```python
from build123d import *

# Parameters (mm, degrees)
SKETCH1_W                  = 600
SKETCH1_H                  = 500
BOSS_EXTRUDE1_DEPTH        = 226
SKETCH2_OUTSIDE_W          = 764.614
SKETCH2_OUTSIDE_H          = 664.614
CUT_EXTRUDE1_DEPTH         = 452.193971591
CUT_EXTRUDE8_DEPTH         = 452.193971591
CUT_EXTRUDE2_DEPTH         = 689.168583997
CUT_EXTRUDE3_DEPTH         = 689.168583997
SKETCH7_R                  = 2.5
CUT_EXTRUDE5_DEPTH         = 25
SKETCH8_R                  = 9.525
CUT_EXTRUDE6_DEPTH         = 35
F_6_0MM_DOWEL_HOLE1_D      = 6
F_6_0MM_DOWEL_HOLE1_DEPTH  = 28.197418143
F_6_0MM_DOWEL_HOLE1_TIP    = 1.802581857
F_6_0MM_DOWEL_HOLE2_D      = 6
F_6_0MM_DOWEL_HOLE2_DEPTH  = 28.197418143
F_6_0MM_DOWEL_HOLE2_TIP    = 1.802581857
F_6_0MM_DOWEL_HOLE3_D      = 6
F_6_0MM_DOWEL_HOLE3_DEPTH  = 28.197418143
F_6_0MM_DOWEL_HOLE3_TIP    = 1.802581857
FILLET2_R                  = 30
F_10_0MM_DOWEL_HOLE1_D     = 10
F_10_0MM_DOWEL_HOLE1_DEPTH = 28
F_10_0MM_DOWEL_HOLE1_TIP   = 3.004303095
CUT_EXTRUDE9_DEPTH         = 35
CHAMFER1_SIZE              = 6
CHAMFER1_SIZE_2            = 114.486820126
CHAMFER2_SIZE              = 3
CHAMFER2_SIZE_2            = 171.477335318
CHAMFER2_SIZE_3            = 42.90199877
CHAMFER3_SIZE              = 3
CHAMFER3_SIZE_2            = 171.477335318
CHAMFER3_SIZE_3            = 42.90199877
FILLET3_R                  = 8


with BuildPart() as part:
    # Sketch1 → Boss-Extrude1 (new body)
    with BuildSketch(Plane.XY):
        Rectangle(SKETCH1_W, SKETCH1_H)
    extrude(amount=BOSS_EXTRUDE1_DEPTH)

    # Sketch2 outside → Cut-Extrude1 (cut, through all)
    with BuildSketch(Plane.XY.offset(226)):
        Rectangle(SKETCH2_OUTSIDE_W, SKETCH2_OUTSIDE_H)
        Polygon((-210, -250), (-210, -225), (-210, -30), (210, -30), (210, -225), (210, -250), (300, -250), (300, 250), (-300, 250), (-300, -250), align=None, mode=Mode.SUBTRACT)
    extrude(amount=-CUT_EXTRUDE1_DEPTH, mode=Mode.SUBTRACT)

    # Sketch22 → Cut-Extrude8 (cut, through all)
    with BuildSketch(Plane.XY.offset(226)):
        Polygon((-210, -30), (210, -30), (105, 5), (0, 5), (-105, 5), align=None)
    extrude(amount=-CUT_EXTRUDE8_DEPTH, mode=Mode.SUBTRACT)

    # Sketch4 → Cut-Extrude2 (cut, through all)
    with BuildSketch(Plane.ZY.offset(300)):
        Polygon((148, 25), (148, 5), (226, -200), (226, -165), (226, -145), (226, 250), (148, 250), align=None)
    extrude(amount=-CUT_EXTRUDE2_DEPTH, mode=Mode.SUBTRACT)

    # Sketch5 → Cut-Extrude3 (cut, through all)
    with BuildSketch(Plane.ZY.offset(300)):
        Polygon((131, 160), (131, 165), (148, 185), (148, 65), (131, 85), (131, 90), (131, 125), align=None)
    extrude(amount=-CUT_EXTRUDE3_DEPTH, mode=Mode.SUBTRACT)

    # Sketch7 → Cut-Extrude5 (cut)
    with BuildSketch(Plane.XY.offset(148)):
        with Locations((-270, 215)):
            Circle(SKETCH7_R)
        with Locations((-210, 215)):
            Circle(SKETCH7_R)
        with Locations((-150, 215)):
            Circle(SKETCH7_R)
        with Locations((-90, 215)):
            Circle(SKETCH7_R)
        with Locations((-30, 215)):
            Circle(SKETCH7_R)
        with Locations((30, 215)):
            Circle(SKETCH7_R)
        with Locations((90, 215)):
            Circle(SKETCH7_R)
        with Locations((150, 215)):
            Circle(SKETCH7_R)
        with Locations((210, 215)):
            Circle(SKETCH7_R)
        with Locations((270, 215)):
            Circle(SKETCH7_R)
        with Locations((-210, 35)):
            Circle(SKETCH7_R)
        with Locations((-150, 35)):
            Circle(SKETCH7_R)
        with Locations((-90, 35)):
            Circle(SKETCH7_R)
        with Locations((-30, 35)):
            Circle(SKETCH7_R)
        with Locations((30, 35)):
            Circle(SKETCH7_R)
        with Locations((90, 35)):
            Circle(SKETCH7_R)
        with Locations((150, 35)):
            Circle(SKETCH7_R)
        with Locations((210, 35)):
            Circle(SKETCH7_R)
        with Locations((270, 35)):
            Circle(SKETCH7_R)
        with Locations((-270, 35)):
            Circle(SKETCH7_R)
    extrude(amount=-CUT_EXTRUDE5_DEPTH, mode=Mode.SUBTRACT)

    # Sketch8 → Cut-Extrude6 (cut)
    with BuildSketch(Plane.XZ.offset(250)):
        with Locations((240, 171)):
            Circle(SKETCH8_R)
        with Locations((275, 171)):
            Circle(SKETCH8_R)
        with Locations((240, 51)):
            Circle(SKETCH8_R)
        with Locations((275, 51)):
            Circle(SKETCH8_R)
        with Locations((-275, 51)):
            Circle(SKETCH8_R)
        with Locations((-240, 51)):
            Circle(SKETCH8_R)
        with Locations((-275, 171)):
            Circle(SKETCH8_R)
        with Locations((-240, 171)):
            Circle(SKETCH8_R)
    extrude(amount=-CUT_EXTRUDE6_DEPTH, mode=Mode.SUBTRACT)

    # Ø6.0mm Dowel Hole1
    with Locations(Plane.ZY.offset(300)):
        with Locations((114, 95), (64, 95), (64, 155), (114, 155), (98, 230), (98, 200), (98, 50), (98, 20), (68, 230), (68, 200), (68, 50), (68, 20)):
            Hole(F_6_0MM_DOWEL_HOLE1_D / 2, depth=F_6_0MM_DOWEL_HOLE1_DEPTH)
            with Locations((0, 0, -(F_6_0MM_DOWEL_HOLE1_DEPTH + F_6_0MM_DOWEL_HOLE1_TIP / 2))):  # 118° drill point
                Cone(0, F_6_0MM_DOWEL_HOLE1_D / 2, F_6_0MM_DOWEL_HOLE1_TIP, mode=Mode.SUBTRACT)

    # Ø6.0mm Dowel Hole2
    with Locations(Plane(origin=(300, 0, 0), x_dir=(0, 0, -1), z_dir=(1, 0, 0))):
        with Locations((-128, 230), (-128, 200), (-114, 155), (-64, 155), (-64, 95), (-114, 95), (-128, 50), (-128, 20)):
            Hole(F_6_0MM_DOWEL_HOLE2_D / 2, depth=F_6_0MM_DOWEL_HOLE2_DEPTH)
            with Locations((0, 0, -(F_6_0MM_DOWEL_HOLE2_DEPTH + F_6_0MM_DOWEL_HOLE2_TIP / 2))):  # 118° drill point
                Cone(0, F_6_0MM_DOWEL_HOLE2_D / 2, F_6_0MM_DOWEL_HOLE2_TIP, mode=Mode.SUBTRACT)

    # Ø6.0mm Dowel Hole3
    with Locations(Plane(origin=(300, 0, 0), x_dir=(0, 0, -1), z_dir=(1, 0, 0))):
        with Locations((-110, 215), (-80, 215), (-50, 215), (-50, 35), (-80, 35), (-110, 35)):
            Hole(F_6_0MM_DOWEL_HOLE3_D / 2, depth=F_6_0MM_DOWEL_HOLE3_DEPTH)
            with Locations((0, 0, -(F_6_0MM_DOWEL_HOLE3_DEPTH + F_6_0MM_DOWEL_HOLE3_TIP / 2))):  # 118° drill point
                Cone(0, F_6_0MM_DOWEL_HOLE3_D / 2, F_6_0MM_DOWEL_HOLE3_TIP, mode=Mode.SUBTRACT)

    # Fillet2
    fillet2_edges = [part.edges().sort_by_distance(p)[0] for p in [
        (210, -30, 80.658536585),
        (-210, -30, 80.658536585),
        (-105, 5, 74),
        (105, 5, 74),
    ]]
    fillet(fillet2_edges, radius=FILLET2_R)

    # Ø10.0mm Dowel Hole1
    with Locations(Plane(origin=(0, 250, 0), x_dir=(1, 0, 0), z_dir=(0, 1, 0))):
        with Locations((-150, -74), (150, -74)):
            Hole(F_10_0MM_DOWEL_HOLE1_D / 2, depth=F_10_0MM_DOWEL_HOLE1_DEPTH)
            with Locations((0, 0, -(F_10_0MM_DOWEL_HOLE1_DEPTH + F_10_0MM_DOWEL_HOLE1_TIP / 2))):  # 118° drill point
                Cone(0, F_10_0MM_DOWEL_HOLE1_D / 2, F_10_0MM_DOWEL_HOLE1_TIP, mode=Mode.SUBTRACT)

    # Sketch10 → Cut-Extrude9 (cut)
    with BuildSketch(Plane(origin=(0, 0, 0), x_dir=(-1, 0, 0), z_dir=(0, 0, -1))):
        Polygon((150, 142), (150, 138), (235, 138), (235, 142), (235, 155), (300, 155), (300, 250), (150, 250), (150, 155), align=None)
    extrude(amount=-CUT_EXTRUDE9_DEPTH, mode=Mode.SUBTRACT)

    # Chamfer1
    # the kernel refuses this chamfer: 114.486820126, 6 mm, written as the material it takes off along each edge
    with BuildSketch(Plane(origin=(-597.650645388, 250, 35), x_dir=(0, 0.5911482838883376, 0.8065628967761121), z_dir=(1, 0, 0))) as chamfer1_piece_1_section:
        Polygon((CHAMFER1_SIZE * 0.806562896776, CHAMFER1_SIZE * 0.591148283888), (-CHAMFER1_SIZE_2 * 0.59114828389, CHAMFER1_SIZE_2 * 0.806562896779), (0, 0), align=None)
    chamfer1_piece_1 = extrude(amount=447.650645388, mode=Mode.PRIVATE)
    chamfer1_piece_1 = split(chamfer1_piece_1, bisect_by=Plane(origin=(-267.5, 155, 37.049515036), z_dir=(0, 1, 0)), keep=Keep.TOP, mode=Mode.PRIVATE)
    add(chamfer1_piece_1, mode=Mode.SUBTRACT)
    with BuildSketch(Plane(origin=(-597.650645388, 250, 35), x_dir=(0, 0.5911482838883376, 0.8065628967761121), z_dir=(1, 0, 0))) as chamfer1_piece_2_section:
        Polygon((CHAMFER1_SIZE * 0.806562896776, CHAMFER1_SIZE * 0.591148283888), (-CHAMFER1_SIZE_2 * 0.59114828389, CHAMFER1_SIZE_2 * 0.806562896779), (0, 0), align=None)
    chamfer1_piece_2 = extrude(amount=447.650645388, mode=Mode.PRIVATE)
    chamfer1_piece_2 = split(chamfer1_piece_2, bisect_by=Plane(origin=(-192.5, 138, 35.345336882), z_dir=(0, 1, 0)), keep=Keep.TOP, mode=Mode.PRIVATE)
    chamfer1_piece_2 = split(chamfer1_piece_2, bisect_by=Plane(origin=(-235, 148.692020353, 35.345336882), z_dir=(1, 0, 0)), keep=Keep.TOP, mode=Mode.PRIVATE)
    add(chamfer1_piece_2, mode=Mode.SUBTRACT)

    # Chamfer2
    # the kernel refuses this chamfer: 171.477335318, 42.90199877, 3 mm, written as the material it adds along each edge
    with BuildSketch(Plane(origin=(-300, 155, 36.021260968), x_dir=(0, 0.4058983906880882, 0.9139182110215444), z_dir=(1, 0, 0))) as chamfer2_piece_1_section:
        Polygon((CHAMFER2_SIZE * 0.453172904552, -CHAMFER2_SIZE * 0.891422637462), (-CHAMFER2_SIZE_2 * 0.913918211021, -CHAMFER2_SIZE_2 * 0.405898390688), (0, 0), align=None)
    chamfer2_piece_1 = extrude(amount=65, mode=Mode.PRIVATE)
    chamfer2_piece_1 = split(chamfer2_piece_1, bisect_by=Plane(origin=(-267.5, 156.347115751, 0), z_dir=(0, 0, 1)), keep=Keep.TOP, mode=Mode.PRIVATE)
    add(chamfer2_piece_1)
    # the kernel refuses this chamfer: 171.477335318, 42.90199877, 3 mm, written as the material it adds along each edge
    with BuildSketch(Plane(origin=(-235, 269.37818115, 42.015567441), x_dir=(0.8766829747338777, -0.025177183236006113, 0.4804092747398407), z_dir=(-1.4194297151346516e-15, -0.9986295347545833, -0.0523359562427643))) as chamfer2_2_piece_1_section:
        Polygon((CHAMFER2_SIZE * 0.876682974734, -CHAMFER2_SIZE * 0.481068562485), (-CHAMFER2_SIZE_3 * 0.481068562487, -CHAMFER2_SIZE_3 * 0.876682974737), (0, 0), align=None)
    chamfer2_2_piece_1 = extrude(amount=243.09362506, mode=Mode.PRIVATE)
    chamfer2_2_piece_1 = split(chamfer2_2_piece_1, bisect_by=Plane(origin=(-233.972430934, 147.892877169, 0), z_dir=(0, 0, 1)), keep=Keep.TOP, mode=Mode.PRIVATE)
    chamfer2_2_piece_1 = split(chamfer2_2_piece_1, bisect_by=Plane(origin=(-233.972430934, 157.747464866, 21.946082382), z_dir=(0, -0.9998476951563882, 0.017452406437459534)), keep=Keep.TOP, mode=Mode.PRIVATE)
    add(chamfer2_2_piece_1)

    # Chamfer3
    # the kernel refuses this chamfer: 171.477335318, 42.90199877, 3 mm, written as the material it adds along each edge
    with BuildSketch(Plane(origin=(-677.838560586, 138, 35.13032872), x_dir=(0, 0.4058983906880882, 0.9139182110215444), z_dir=(1, 0, 0))) as chamfer3_piece_1_section:
        Polygon((CHAMFER3_SIZE * 0.453172904552, -CHAMFER3_SIZE * 0.891422637462), (-CHAMFER3_SIZE_2 * 0.913918211021, -CHAMFER3_SIZE_2 * 0.405898390688), (0, 0), align=None)
    chamfer3_piece_1 = extrude(amount=973.677121172, mode=Mode.PRIVATE)
    chamfer3_piece_1 = split(chamfer3_piece_1, bisect_by=Plane(origin=(-300, 139.34996863, 18.189156811), z_dir=(1, 0, 0)), keep=Keep.TOP, mode=Mode.PRIVATE)
    chamfer3_piece_1 = split(chamfer3_piece_1, bisect_by=Plane(origin=(-191.593979547, 139.34996863, 0), z_dir=(0, 0, 1)), keep=Keep.TOP, mode=Mode.PRIVATE)
    add(chamfer3_piece_1)
    # the kernel refuses this chamfer: 171.477335318, 42.90199877, 3 mm, written as the material it adds along each edge
    with BuildSketch(Plane(origin=(-150, 29.613596059, 29.450037985), x_dir=(-0.8766829747338778, -0.025177183236005013, 0.4804092747398405), z_dir=(0, 0.9986295347545833, 0.052335956242764624))) as chamfer3_2_piece_1_section:
        Polygon((CHAMFER3_SIZE * 0.876682974734, -CHAMFER3_SIZE * 0.481068562485), (-CHAMFER3_SIZE_3 * 0.481068562487, -CHAMFER3_SIZE_3 * 0.876682974737), (0, 0), align=None)
    chamfer3_2_piece_1 = extrude(amount=332.223997929, mode=Mode.PRIVATE)
    chamfer3_2_piece_1 = split(chamfer3_2_piece_1, bisect_by=Plane(origin=(-151.011869229, 250, 24.17159315), z_dir=(0, -1, 0)), keep=Keep.TOP, mode=Mode.PRIVATE)
    chamfer3_2_piece_1 = split(chamfer3_2_piece_1, bisect_by=Plane(origin=(-151.011869229, 195.655839269, 0), z_dir=(0, 0, 1)), keep=Keep.TOP, mode=Mode.PRIVATE)
    add(chamfer3_2_piece_1)

    # Fillet3
    fillet3_edges = [part.edges().sort_by_distance(p)[0] for p in [
        (-233.262026443, 157.680141588, 18.089134418),
        (-233.230947563, 140.687917229, 17.643668295),
        (-151.769052437, 140.687917229, 17.643668295),
    ]]
    fillet(fillet3_edges, radius=FILLET3_R)


solid = part.part
```
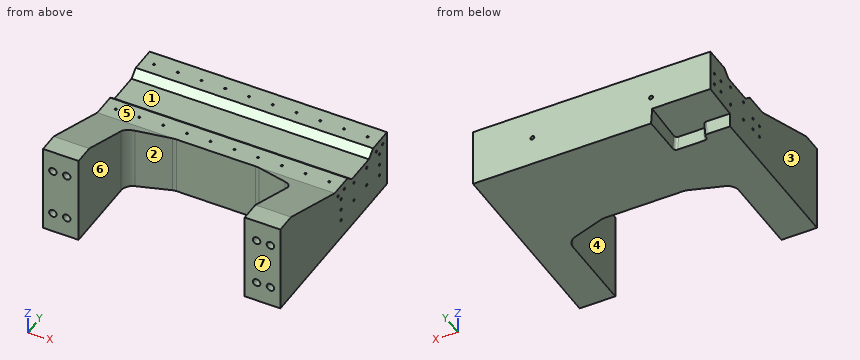
Read the model definition and answer for the solid it produces. Units are mm, in the model's axes. Face numbers are marked on the shaded views. A direction names the side the tool comes from. Give positions to 0.01 mm unless a question says otherwise; leave off trailing zeros. Order: outer loops, then holes, each group sorted by start corner. A loop starts at its lowest first (then second) coordinate and runs counter-clockwise, first axis right, second up.
(1) For a pull along X with two mould halves and no side action, classify the marked faces 1, 2, 3 and 4 as released by +X, released by -X, zero draft, split by the parting line, or undercut.
(2) Find section C-C (y = 128). Give the vertices of the cut face in (x, z), plus the area to 3 significant figures.
(3) Given pin 1 (5.5 mm diameter, centred on x = 210.5, y = 214.5, fed in from +Z); pin 2 (6 mm diameter, centred on x = -117.5, y = 167.5, fed in from +Z) (3 decimals); pin 3 (9.5 mm diameter, centred on x = 276, z = 47, fed in from -Y); pin 4 (4 mm diameter, centred on x = -30, y = 35, fed in from -Z), each flat-ended and moving along its own axis, determine where each tip first touches the part or whether it passes through.
(4) For the marked faces 5, 6 and 7, determine the directions among +Z, -Z, +X, -X, +Y, -Y from which every point of the face is accessible in a straight line to the end or side of a thin tool.
(5) Straight lines are drawn through the part: L1, parallel to Y at x = -282, z = 98; L2, parallel to Z at x = -240, y = -225.5 (3 decimals); L3, parallel to Z at x = 291, y = 95. For each, find the intervals that lie inside material, in ascending order.
(6) Find section D-D (y = -69.5). Give the vertices of the cut face in (x, z).
(7) Find section B-B (y = -146.5). Give the vertices of the cut face in (x, z), plus the area to 3 significant figures.
(8) Find section A-A (x = 240). Give the vertices of the cut face in (y, z) (3 decimals).
Result sheet:
1. face 1: zero draft
1. face 2: undercut
1. face 3: released by -X
1. face 4: undercut
2. outline: (-300, 0) - (300, 0) - (300, 131) - (-300, 131) - close
2. area: 78,600 mm2
3. pin 1: stops at z = 148
3. pin 2: stops at z = 135.675
3. pin 3: stops at y = -215
3. pin 4: stops at z = 0
4. face 5: +Z, +X, -X, +Y
4. face 6: +Z, -Z, -Y
4. face 7: +Z, -Z, +X, -X, -Y
5. L1: y = -250 to 17, 23 to 47, 53 to 197, 203 to 227, 233 to 250
5. L2: z = 0 to 41.475, 60.525 to 161.475, 180.525 to 226
5. L3: z = 0 to 61, 67 to 111, 117 to 131
6. outline: (-300, 0) - (-210, 0) - (-210, 176.35) - (-300, 176.35) - close; (210, 0) - (300, 0) - (300, 176.35) - (210, 176.35) - close
7. outline: (-300, 0) - (-210, 0) - (-210, 205.64) - (-300, 205.64) - close; (210, 0) - (300, 0) - (300, 205.64) - (210, 205.64) - close
7. area: 37,000 mm2
8. outline: (-250, 0) - (250, 0) - (250, 148) - (185, 148) - (165, 131) - (85, 131) - (65, 148) - (5, 148) - (-200, 226) - (-250, 226) - (-250, 180.525) - (-215, 180.525) - (-215, 161.475) - (-250, 161.475) - (-250, 60.525) - (-215, 60.525) - (-215, 41.475) - (-250, 41.475) - close
